Autodesk Inventor part; units mm, degrees
ref_plane "YZ Plane" through (0, 0, 0) normal (1, 0, 0) x (0, 1, 0)
ref_plane "XZ Plane" through (0, 0, 0) normal (0, 1, 0) x (-1, 0, 0)
ref_plane "XY Plane" through (0, 0, 0) normal (0, 0, 1) x (1, 0, 0)
sketch "スケッチ1" plane through (0, 0, 0) normal (0, 0, 1) x (1, 0, 0)
  circle A0 centre (0, 0) radius 4
  dimension "d13" = 8
extrude "押し出し1" add sketch "スケッチ1" along normal mid plane 40
sketch "スケッチ2" plane through (0, 0, 20) normal (0, 0, 1) x (1, 0, 0)
  point P0 (0, 0)
  point P1 (0, 0)
hole "穴1" at (0, 0, 20) direction (0, 0, -1) diameter 3.242 depth 11.8 tip angle 118
mirror "ミラー1" about plane through (0, 0, 0) normal (0, 0, 1) of "穴1"
chamfer "面取り1" distance 0.2 angle 45 4 edges at (0, 1.621, 20) (-4, 0, 20) (-4, 0, -20) (0, 1.621, -20)
properties part number "unir-spacer5" material "鋼、炭素鋼"
The listing builds one solid part. Answer for the finished solid, in the listing's coordinates (mm). A direction names the side the tool comes from. Coordinates: 2 decimals unless noted, no trailing zeros. Write each loop counter-clockwise with the first axis right and the second up, starting at its lowest first coordinate (ties: lowest second). Pieces come first, ordered by that corner, then holes. Notation, with made-up numbers: (14, 49) - (59, 49) arc R18 cw to (59, 81) - close; hole circle Ø11 at (-27.75, -31). An arc over 180 degrees is marked (long way). One line per item, written item: value.
1) A tool of negligible diameter and unlimited length cuts with its end or side. For faces 4 (the cylindrical face through (1.438, -0.748, 13.919)), 5 (the flat face through (2, 1, -20)), from which of +Z, -Z, +X, -X, +Y, -Y can it reach the whole face along a straight path? Write none if from no direction.
Geometry check:
face 4: +Z
face 5: -Z, +X, -X, +Y, -Y
2) Each of these flat-tipped pins is pushed along its axis until it touches: pin 1 Ø1.9 at (x, y) = (0, 0) entering from -Z; pin 2 Ø1 at (x, z) = (2, 14.5) entering from +Y; pin 3 Ø1.9 at (x, y) = (0, 0) entering from +Z. Where does it stop, or does it pass through?
Geometry check:
pin 1: stops at z = -7.8
pin 2: stops at y = 3.71
pin 3: stops at z = 7.8
3) For a pull along X with two mould halves and no side action, classify faces 1 (the cylindrical face through (-1.438, -0.748, -13.919)), 2 (the flat face through (2, 1, 20)), 3 (the cylindrical face through (-0.867, 3.905, -0.277)) as pulls with the +X half, pulls with the -X half, needs draft (parallel to the pull), parting line crosses it, or undercut.
Geometry check:
face 1: undercut
face 2: needs draft
face 3: parting line crosses it
4) Find section B-B (z = -0.5). Give the vertices of the cut face in (x, y).
Geometry check:
outline: circle Ø8 at (0, 0)
5) Find section A-A (z = -13). Give the vertices of the cut face in (x, y), and give its area (3 significant figures).
Geometry check:
outline: circle Ø8 at (0, 0); hole circle Ø3.24 at (0, 0)
area: 42.0 mm2
6) Consider line 1 along Y through (x, z) = (0, 11.75); line 2 along Y through (x, z) = (1.25, -9); line 3 along Z through (x, y) = (-0.5, 1). Determine where each line is inside the solid, lowest interval first. Write a range as from..to.
Geometry check:
line 1: y = -4..-1.62, 1.62..4
line 2: y = -3.8..-1.03, 1.03..3.8
line 3: z = -7.9..7.9
